```python
from build123d import *

# Parameters (mm, degrees)
SCHIZZO1_R                   = 10
ESTRUSIONE_ESTRUSIONE1_DEPTH = 10
SCHIZZO2_R                   = 3
ESTRUSIONE_ESTRUSIONE2_DEPTH = 3.2
SMUSSO1_SIZE                 = 0.5


with BuildPart() as part:
    # Schizzo1 → Estrusione-Estrusione1 (new, symmetric)
    with BuildSketch(Plane(origin=(0, 0, 0), x_dir=(1, 0, 0), z_dir=(0, 1, 0))):
        with Locations(Location((0, 0, 0), (0, 0, 270))):
            Circle(SCHIZZO1_R)
    extrude(amount=ESTRUSIONE_ESTRUSIONE1_DEPTH, both=True)

    # Schizzo2 → Estrusione-Estrusione2 (add)
    with BuildSketch(Plane.XZ.offset(10)):
        with Locations(Location((0, 0, 0), (0, 0, 270))):
            Circle(SCHIZZO2_R)
    estrusione_estrusione2 = extrude(amount=ESTRUSIONE_ESTRUSIONE2_DEPTH)

    # Specchia1: Estrusione-Estrusione2 across plane
    add(estrusione_estrusione2.mirror(Plane.ZX))

    # Schizzo8 → Foro per Vite M10-1 (revolve, cut)
    with BuildSketch(Plane(origin=(0, 0, 10), x_dir=(0, -1, 0), z_dir=(1, 0, 0))):
        Polygon((0, 0), (0, 20), (5.5, 20), (5.5, 0.025), (5.525, 0), align=None)
    revolve(axis=Axis((0, 0, 16.35), (0, 0, -1)), mode=Mode.SUBTRACT)

    # Smusso1
    smusso1_edges = [part.edges().sort_by_distance(p)[0] for p in [
        (0, 13.2, 3),
        (0, -13.2, 3),
    ]]
    chamfer(smusso1_edges, length=SMUSSO1_SIZE)


solid = part.part
```
Can you work these out from the model? Positions are in its coordinate system, mm. A direction names the side the tool comes from. Round coordinates to 2 decimals unless told otherwise and drop trailing zeros. Loops run counter-clockwise (first coordinate to the right, second up) from the corner with the lowest first, then second, coordinate; pieces in that order, holes last. Notation, with made-up numbers: M 14.25,39.5 L 45.25,39.5 A12 ccw 45.25,45.5 Z; hole C -31.5,-39.5 d10. An arc over 180 degrees is marked long. Write item = value, one per line. Start each with the question number.
(1) If we mould it in two halves opening along X, with no side actions, what happens to faces 4 (the face through (2.4, -10, 2.1)), 5 (the face through (-3.72, 4.05, 0.13)), 6 (the face through (-6, 0, -8))? For each: released by +X, released by -X, zero draft, split by the parting line, or undercut.
(2) Suppose I cut it at B-B on z = 0. Write out the boundary of the cut face in (x, y), plus the area to 3 significant figures.
(3) Suppose I cut it at C-C on y = -7.75. Write out the boundary of the cut face in (x, z).
(4) Suppose I cut it at A-A on x = 0. Write out the boundary of the cut face in (y, z) (3 decimals).
(5) Suppose I cut it at D-D on y = 0. Write out the boundary of the cut face in (x, z).
(6) I'm going to push flat-ended pins straight in: P1, Ø10, axis at x = 3.5, z = 1, coming from the -Y side; P2, Ø2, axis at x = -1, y = 3, coming from the -Z side (1 decimal); P3, Ø6, axis at x = -3.5, y = -9.5, coming from the +Z side; P4, Ø4, axis at x = -4, z = -6.5, coming from the -Y side. Where does each tip first touch, or does it pass through?
(7) I need wall thicknesses on line 1 along Y through (x, z) = (0, 4.25); line 2 along X through (y, z) = (-2.5, 8.5). Which ranges of each line are inside material? Lowest first, please.
(8) Which directions (+Z, -Z, +X, -X, +Y, -Y) give clear straight access to the entire face, cutting with the end or side of a thin tool? Please do faces 1 (the face through (0, 13.2, 0)), 2 (the face through (0.9, -11.33, -2.86)), 3 (the face through (2.4, 10, 2.1)).
Answer block:
q1.face_4 = zero draft
q1.face_5 = undercut
q1.face_6 = split by the parting line
q2.outline = M -10,-10 L -3,-10 L -3,-12.7 L -2.5,-13.2 L 2.5,-13.2 L 3,-12.7 L 3,-10 L 10,-10 L 10,10 L 3,10 L 3,12.7 L 2.5,13.2 L -2.5,13.2 L -3,12.7 L -3,10 L -10,10 Z; hole C 0,0 d11
q2.area = 343 mm²
q3.outline = C 0,0 d20
q4.outline = M -13.2,-2.5 L -12.7,-3 L -10,-3 L -10,-10 L -5.5,-10 L -5.5,9.975 L -5.525,10 L -10,10 L -10,3 L -12.7,3 L -13.2,2.5 Z; M 5.5,-10 L 10,-10 L 10,-3 L 12.7,-3 L 13.2,-2.5 L 13.2,2.5 L 12.7,3 L 10,3 L 10,10 L 5.525,10 L 5.5,9.975 Z
q5.outline = M -5.5,-8.35 L -5.5,8.35 A10 ccw Z; M 5.5,-8.35 A10 ccw 5.5,8.35 Z
q6.P1 = -13.2
q6.P2 = through
q6.P3 = 9.99
q6.P4 = -10
q7.line_1 = -10 to -5.5, 5.5 to 10
q7.line_2 = -5.27 to -4.9, 4.9 to 5.27
q8.face_1 = +Z, -Z, +X, -X, +Y
q8.face_2 = -Y
q8.face_3 = +Y
